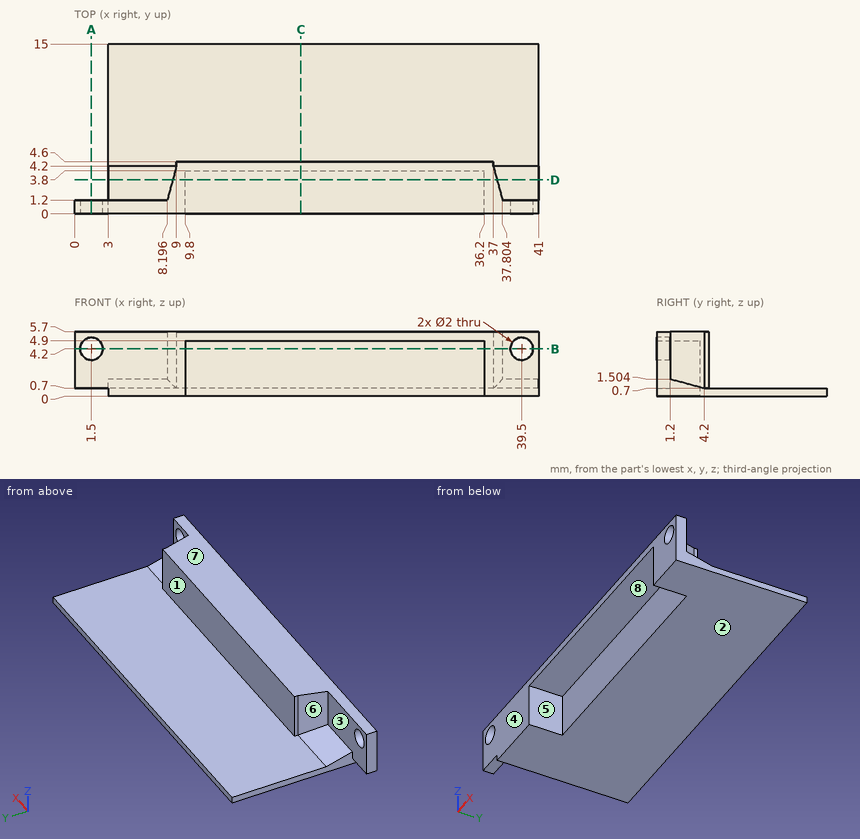
Could you check a few things on this drawing? It's one solid part, dimensions in mm from its lowest x, y, z. A direction names the side the tool comes from. Coordinates: 2 decimals unless noted, no trailing zeros. Order: outer loops, then holes, each group sorted by start corner. A loop starts at its lowest first (then second) coordinate and runs counter-clockwise, first axis right, second up. Notation, with made-up numbers: (35.25, -3) -> (57.25, -3) arc R29 cw to (57.25, 29) -> close; hole circle Ø6 at (10.25, 63). An arc over 180 degrees is marked (long way). Answer in a Markdown table with one row per item.
(1) I want a section at C-C on x = 20. List the corners of the cut face in (y, z) for me.
Answer key:
| item | result |
|---|---|
| outline | (0, 4.9) -> (3.8, 4.9) -> (3.8, 0) -> (15, 0) -> (15, 0.7) -> (4.6, 0.7) -> (4.6, 5.7) -> (0, 5.7) -> close |
(2) I want a section at A-A on x = 1.5. List the corners of the cut face in (y, z) for me, then the cut area to 3 significant figures.
Answer key:
| item | result |
|---|---|
| outline | (0, 0.7) -> (1.2, 0.7) -> (1.2, 3.2) -> (0, 3.2) -> close; (0, 5.2) -> (1.2, 5.2) -> (1.2, 5.7) -> (0, 5.7) -> close |
| area | 3.60 mm^2 |
(3) I want a section at B-B on z = 4.2. List the corners of the cut face in (x, y) for me, then the cut area to 3 significant figures.
Answer key:
| item | result |
|---|---|
| outline | (0, 0) -> (0.5, 0) -> (0.5, 1.2) -> (0, 1.2) -> close; (2.5, 0) -> (9.8, 0) -> (9.8, 3.8) -> (36.2, 3.8) -> (36.2, 0) -> (38.5, 0) -> (38.5, 1.2) -> (37.8, 1.2) -> (37, 4.2) -> (37, 4.6) -> (9, 4.6) -> (9, 4.2) -> (8.2, 1.2) -> (2.5, 1.2) -> close; (40.5, 0) -> (41, 0) -> (41, 1.2) -> (40.5, 1.2) -> close |
| area | 41.7 mm^2 |
(4) I want a section at D-D on y = 3. List the corners of the cut face in (x, z) for me.
Answer key:
| item | result |
|---|---|
| outline | (3, 0) -> (9.8, 0) -> (9.8, 4.9) -> (36.2, 4.9) -> (36.2, 0) -> (41, 0) -> (41, 1.02) -> (37.32, 1.02) -> (37.32, 5.7) -> (8.68, 5.7) -> (8.68, 1.02) -> (3, 1.02) -> close |
(5) On a 3-axis mill with a long thin cutter (end or side, diameter ignored), from which of +Z, -Z, +X, -X, +Y, -Y can I reach the whole of each face in a straight line? I mean the marked faces 1, 2, 3, 4 and 5. Say none if no direction works.
Answer key:
| item | result |
|---|---|
| face 1 | +Z, +X, -X, +Y |
| face 2 | -Z, +X, -X, +Y, -Y |
| face 3 | +Z, -X, +Y |
| face 4 | +Z, -Z, +X, -X, -Y |
| face 5 | -Z, -Y |
(6) Please list where these lines run through material, in increasing order: probe 1 along X at (y, z) = (0.85, 4.2); probe 2 along Z at (x, y) = (39.5, 0.3); probe 3 along Z at (x, y) = (1.5, 1).
Answer key:
| item | result |
|---|---|
| probe 1 | 0 to 0.5, 2.5 to 9.8, 36.2 to 38.5, 40.5 to 41 |
| probe 2 | 0 to 3.2, 5.2 to 5.7 |
| probe 3 | 0.7 to 3.2, 5.2 to 5.7 |
(7) Will these pins go through, and if not, where does the flat tip stop? pin 1 Ø1.9 at (x, y) = (16.5, 2.5) entering from -Z; pin 2 Ø1.5 at (y, z) = (3.5, 1.5) entering from -X; pin 3 Ø0.6 at (x, y) = (1, 0.5) entering from -Z.
Answer key:
| item | result |
|---|---|
| pin 1 | z = 4.9 |
| pin 2 | x = 3 |
| pin 3 | z = 0.7 |
(8) Thinking about a two-plate mould opening in X: for the marked faces 6, 7 and 8, which applies, +X half, -X half, draft (parallel to the pull), parting line (faces both ways), or undercut?
Answer key:
| item | result |
|---|---|
| face 6 | -X half |
| face 7 | draft |
| face 8 | undercut |
